Build history of the part. All positions in model axes, mm. A direction names the side the tool comes from. Give positions to 0.01 mm unless a question says otherwise; leave off trailing zeros. Loops run counter-clockwise (first coordinate to the right, second up) from the corner with the lowest first, then second, coordinate; pieces in that order, holes last. Notation, with made-up numbers: (-38, -22.75) -> (16, -22.75) arc R21 ccw to (16, -2.75) -> close; hole circle Ø4 at (74, 55). An arc over 180 degrees is marked (long way). Answer as a JSON object with one key per item and string values. Group by question number.
from build123d import *

# Parameters (mm, degrees)
SKETCH2_W           = 38.1
SKETCH2_H           = 17.78
BOSS_EXTRUDE1_DEPTH = 8.89
SKETCH3_W           = 38.1
SKETCH3_H           = 8.763
BOSS_EXTRUDE2_DEPTH = 25.4
SKETCH4_R           = 1.524
CUT_EXTRUDE1_DEPTH  = 44.067795393
FILLET1_R           = 1.27


with BuildPart() as part:
    # Sketch2 → Boss-Extrude1 (new body)
    with BuildSketch(Plane(origin=(0, 0, 0), x_dir=(1, 0, 0), z_dir=(0, 1, 0))):
        Rectangle(SKETCH2_W, SKETCH2_H)
    extrude(amount=BOSS_EXTRUDE1_DEPTH)

    # Sketch3 → Boss-Extrude2 (add)
    with BuildSketch(Plane(origin=(0, 8.89, 0), x_dir=(1, 0, 0), z_dir=(0, 1, 0))):
        with Locations((0, 4.5085)):
            Rectangle(SKETCH3_W, SKETCH3_H)
    extrude(amount=BOSS_EXTRUDE2_DEPTH)

    # Sketch4 → Cut-Extrude1 (cut, through all)
    with BuildSketch(Plane.XY.offset(8.89)):
        with Locations((-10.16, 4.445)):
            Circle(SKETCH4_R)
        with Locations((10.16, 4.445)):
            Circle(SKETCH4_R)
    extrude(amount=-CUT_EXTRUDE1_DEPTH, mode=Mode.SUBTRACT)

    # Fillet1
    fillet1_edges = [part.edges().sort_by_distance(p)[0] for p in [
        (0, 34.29, -8.89),
        (0, 0, -8.89),
        (-19.05, 17.145, -8.89),
        (19.05, 17.145, -8.89),
    ]]
    fillet(fillet1_edges, radius=FILLET1_R)


solid = part.part
(1) 3-axis set-ups, long thin cutter, end or side, ignore diameter. For faces 4 (the flat face through (0, 21, -0.127)), 5 (the cylindrical face through (-11.683, 4.512, 0.124)): which of +Z, -Z, +X, -X, +Y, -Y reach the whole face in a straight line?
(2) Pull direction X, two halves, no side cores. Call faces 1 (the cylindrical face through (18.668, 16.905, -8.528)), 2 (the cylindrical face through (8.637, 4.512, 0.124)), 3 (the flat face through (0, 4, 8.89)): pulls with the +X half, pulls with the -X half, needs draft (parallel to the pull), parting line crosses it, or undercut.
(3) Saw through at A-A on x = -10.16. List the corners of the cut face in (y, z).
(4) Pin check, flat tips, straight feed: pin 1 (5 mm diameter, centred on x = 10.16, y = 4.445, fed in from -Z); pin 2 (2.5 mm diameter, centred on x = 1.5, z = 4.5, fed in from +Y). Stop position of each tip, or through.
(5) Saw through at B-B on y = 4. List the corners of the cut face in (x, z), plus the area to 3 significant figures.
(6) Saw through at C-C on x = 1. List the corners of the cut face in (y, z), plus the area to 3 significant figures.
(7) Probe line 1 along Y through (x, z) = (10.16, -5); line 2 along X through (y, z) = (4.5, 2.25); line 3 along Y through (x, z) = (10.16, 0.5). List the from-to ranges inside material, lowest first. Write a range as [from, to].
(8) Saw through at D-D on z = 6.5. List the corners of the cut face in (x, y) (3 decimals).
Calculated:
{
 "1": {"face 4": "+Z, +X, -X, +Y", "face 5": "+Z, -Z"},
 "2": {"face 1": "pulls with the +X half", "face 2": "undercut", "face 3": "needs draft"},
 "3": {"outline": "(0, -7.62) arc R1.27 ccw to (1.27, -8.89) -> (2.92, -8.89) -> (2.92, 8.89) -> (0, 8.89) -> close; (5.97, -8.89) -> (33.02, -8.89) arc R1.27 ccw to (34.29, -7.62) -> (34.29, -0.13) -> (8.89, -0.13) -> (8.89, 8.89) -> (5.97, 8.89) -> close"},
 "4": {"pin 1": "stops at z = -8.89", "pin 2": "stops at y = 8.89"},
 "5": {"outline": "(-19.05, -7.62) arc R1.27 ccw to (-17.78, -8.89) -> (-11.62, -8.89) -> (-11.62, 8.89) -> (-19.05, 8.89) -> close; (-8.7, -8.89) -> (8.7, -8.89) -> (8.7, 8.89) -> (-8.7, 8.89) -> close; (11.62, -8.89) -> (17.78, -8.89) arc R1.27 ccw to (19.05, -7.62) -> (19.05, 8.89) -> (11.62, 8.89) -> close", "area": "573 mm^2"},
 "6": {"outline": "(0, -7.62) arc R1.27 ccw to (1.27, -8.89) -> (33.02, -8.89) arc R1.27 ccw to (34.29, -7.62) -> (34.29, -0.13) -> (8.89, -0.13) -> (8.89, 8.89) -> (0, 8.89) -> close", "area": "380 mm^2"},
 "7": {"line 1": "y = [0, 2.92], [5.97, 34.29]", "line 2": "x = [-19.05, -11.68], [-8.64, 8.64], [11.68, 19.05]", "line 3": "y = [0, 2.92], [5.97, 8.89]"},
 "8": {"outline": "(-19.05, 0) -> (19.05, 0) -> (19.05, 8.89) -> (-19.05, 8.89) -> close; hole circle Ø3.048 at (-10.16, 4.445); hole circle Ø3.048 at (10.16, 4.445)"}
}
